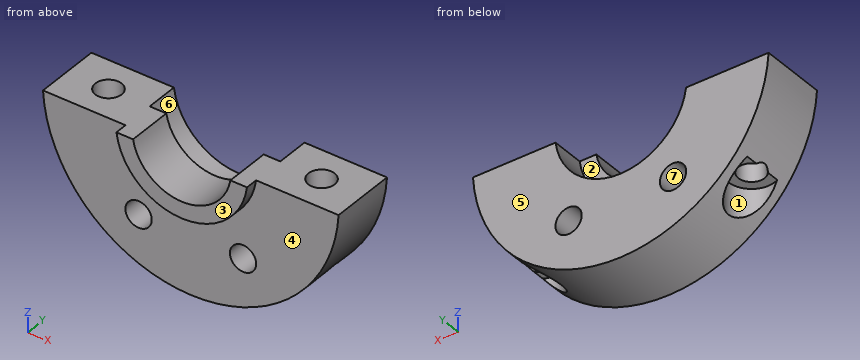
```python
from build123d import *

# Parameters (mm, degrees)
SKETCH1_R           = 18
SKETCH1_R_2         = 8
SKETCH1_R_3         = 1.6
BOSS_EXTRUDE1_DEPTH = 8
SKETCH2_R           = 8
SKETCH2_R_2         = 6
BOSS_EXTRUDE2_DEPTH = 5.5
SKETCH3_W           = 40
SKETCH3_H           = 20
CUT_EXTRUDE1_DEPTH  = 10.5
CUT_EXTRUDE2_REACH  = 19
SKETCH5_R           = 1.6
CUT_EXTRUDE3_REACH  = 29
CUT_EXTRUDE3_START  = -10
SKETCH6_R           = 2.8


with BuildPart() as part:
    # Sketch1 → Boss-Extrude1 (new body)
    with BuildSketch(Plane(origin=(0, 0, 0), x_dir=(1, 0, 0), z_dir=(0, 1, 0))):
        Circle(SKETCH1_R)
        Circle(SKETCH1_R_2, mode=Mode.SUBTRACT)
        with Locations((-6.350852961, 11)):
            Circle(SKETCH1_R_3, mode=Mode.SUBTRACT)
        with Locations((6.350852961, 11)):
            Circle(SKETCH1_R_3, mode=Mode.SUBTRACT)
    extrude(amount=BOSS_EXTRUDE1_DEPTH)

    # Sketch2 → Boss-Extrude2 (add)
    with BuildSketch(Plane(origin=(0, 4, 0), x_dir=(1, 0, 0), z_dir=(0, 1, 0))):
        Circle(SKETCH2_R)
        Circle(SKETCH2_R_2, mode=Mode.SUBTRACT)
    extrude(amount=-BOSS_EXTRUDE2_DEPTH)

    # Sketch3 → Cut-Extrude1 (cut, through all)
    with BuildSketch(Plane(origin=(0, 8, 0), x_dir=(1, 0, 0), z_dir=(0, 1, 0))):
        with Locations((0, -9)):
            Rectangle(SKETCH3_W, SKETCH3_H)
    extrude(amount=-CUT_EXTRUDE1_DEPTH, mode=Mode.SUBTRACT)

    # Sketch5 → Cut-Extrude2 (cut, up to next)
    with BuildSketch(Plane.XY.offset(-1), mode=Mode.PRIVATE) as cut_extrude2_sk1:
        with Locations((-12.954727344, 4)):
            Circle(SKETCH5_R)
    cut_extrude2_tool1 = extrude(cut_extrude2_sk1.sketch, amount=-CUT_EXTRUDE2_REACH, mode=Mode.PRIVATE) & part.part
    add(cut_extrude2_tool1.solids().sort_by_distance((-12.954727, 4, -1))[0], mode=Mode.SUBTRACT)
    # Sketch5 → Cut-Extrude2 (cut, up to next)
    with BuildSketch(Plane.XY.offset(-1), mode=Mode.PRIVATE) as cut_extrude2_sk2:
        with Locations((12.954727344, 4)):
            Circle(SKETCH5_R)
    cut_extrude2_tool2 = extrude(cut_extrude2_sk2.sketch, amount=-CUT_EXTRUDE2_REACH, mode=Mode.PRIVATE) & part.part
    add(cut_extrude2_tool2.solids().sort_by_distance((12.954727, 4, -1))[0], mode=Mode.SUBTRACT)

    # Sketch6 → Cut-Extrude3 (cut, up to next)
    with BuildSketch(Plane.XY.offset(-1).offset(CUT_EXTRUDE3_START), mode=Mode.PRIVATE) as cut_extrude3_sk1:
        with Locations((-12.954727344, 4)):
            Circle(SKETCH6_R)
    cut_extrude3_tool1 = extrude(cut_extrude3_sk1.sketch, amount=-CUT_EXTRUDE3_REACH, mode=Mode.PRIVATE) & part.part
    add(cut_extrude3_tool1.solids().sort_by_distance((-12.954727, 4, -11))[0], mode=Mode.SUBTRACT)
    # Sketch6 → Cut-Extrude3 (cut, up to next)
    with BuildSketch(Plane.XY.offset(-1).offset(CUT_EXTRUDE3_START), mode=Mode.PRIVATE) as cut_extrude3_sk2:
        with Locations((12.954727344, 4)):
            Circle(SKETCH6_R)
    cut_extrude3_tool2 = extrude(cut_extrude3_sk2.sketch, amount=-CUT_EXTRUDE3_REACH, mode=Mode.PRIVATE) & part.part
    add(cut_extrude3_tool2.solids().sort_by_distance((12.954727, 4, -11))[0], mode=Mode.SUBTRACT)


solid = part.part
```
The listing builds one solid part. Answer for the finished solid, in the listing's coordinates (mm). Face numbers are marked on the shaded views. A direction names the side the tool comes from. Round coordinates to 2 decimals unless told otherwise and drop trailing zeros. Order: outer loops, then holes, each group sorted by start corner. A loop starts at its lowest first (then second) coordinate and runs counter-clockwise, first axis right, second up. Notation, with made-up numbers: (14, 40.25) - (18, 40.25) arc R19 cw to (18, 68.25) - close; hole circle Ø5 at (52, -4). An arc over 180 degrees is marked (long way). Put each result on its own line as item: value. Start each with the question number.
(1) Given P1, Ø3, axis at x = 8.5, z = -7, coming from the -Y side; P2, Ø1, axis at y = 1.5, z = -13.5, coming from the -X side; P3, Ø5, axis at y = 2.5, z = -8, coming from the +X side, each flat-ended and moving along its own axis, determine where each tip first touches the part or whether it passes through.
(2) Find section B-B (y = 0.75). Give the vertices of the cut face in (x, z), plus the area to 3 significant figures.
(3) Determine the mould class of the marked faces 5, 6 and 7 for opening direction Z: released by +Z, released by -Z, zero draft, split by the parting line, or undercut.
(4) Find section A-A (z = -10). Give the vertices of the cut face in (x, y), plus the area to 3 significant figures.
(5) For the marked faces 1, 2, 3 and 4, determine the directions among +Z, -Z, +X, -X, +Y, -Y from which every point of the face is accessible in a straight line to the end or side of a thin tool.
(6) Straight lines are drawn through the part: probe 1 along X at (y, z) = (4, -11.9); probe 2 along Y at (x, z) = (-13, -9.25); probe 3 along Y at (x, z) = (11.5, -13.5). For each, find the intervals that lie inside material, in ascending order. Write a range as from..to.
(7) Find section D-D (x = 12). Give the vertices of the cut face in (y, z).
(8) Find section C-C (x = 1). Give the vertices of the cut face in (y, z).
Reply:
1. P1: y = 0
1. P2: x = -12.38
1. P3: x = 17.14
2. outline: (-17.97, -1) arc R18 ccw to (17.97, -1) - (5.92, -1) arc R6 cw to (-5.92, -1) - close; hole circle Ø3.2 at (-6.35, -11); hole circle Ø3.2 at (6.35, -11)
2. area: 412 mm^2
3. face 5: zero draft
3. face 6: released by +Z
3. face 7: undercut
4. outline: (-14.97, 0) - (-7.6, 0) - (-7.6, 8) - (-14.97, 8) - close; (-5.1, 0) - (5.1, 0) - (5.1, 8) - (-5.1, 8) - close; (7.6, 0) - (14.97, 0) - (14.97, 8) - (7.6, 8) - close; hole circle Ø3.2 at (-12.95, 4); hole circle Ø3.2 at (12.95, 4)
4. area: 183 mm^2
5. face 1: -Z
5. face 2: +Z, +Y
5. face 3: +Z, -Z, +X, -X, -Y
5. face 4: -Z, -Y
6. probe 1: -10.15..-7.67, -5.03..5.03, 7.67..10.15
6. probe 2: 0..2.4, 5.6..8
6. probe 3: 0..1.61, 6.39..8
7. outline: (0, -13.42) - (1.37, -13.42) - (1.37, -11) - (2.72, -11) - (2.72, -1) - (0, -1) - close; (5.28, -11) - (6.63, -11) - (6.63, -13.42) - (8, -13.42) - (8, -1) - (5.28, -1) - close
8. outline: (-1.5, -7.94) - (0, -7.94) - (0, -17.97) - (8, -17.97) - (8, -7.94) - (4, -7.94) - (4, -5.92) - (-1.5, -5.92) - close
